Here's the drawing with two shaded views (mm, measured from the low corner). I have some questions. Coordinates: 2 decimals unless noted, no trailing zeros. Write each loop counter-clockwise with the first axis right and the second up, starting at its lowest first coordinate (ties: lowest second). Pieces come first, ordered by that corner, then holes. Notation, with made-up numbers: (42, 13) -> (99, 13) arc R26 ccw to (99, 27) -> close; hole circle Ø9 at (85.5, -2.5). An arc over 180 degrees is marked (long way). Use one line per item in the form item = value.
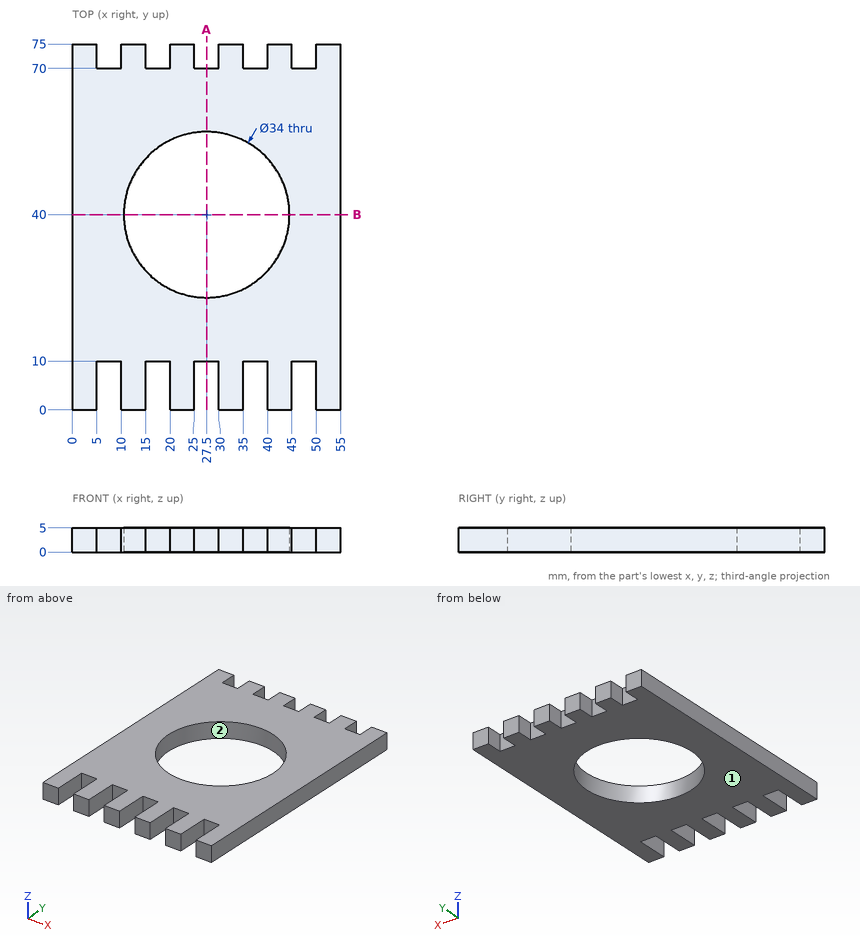
Q1. Suppose I cut it at B-B (y = 40). Write out the boundary of the cut face in (x, z), then the cut area to 3 significant figures.
Return value:
outline = (0, 0) -> (10.5, 0) -> (10.5, 5) -> (0, 5) -> close; (44.5, 0) -> (55, 0) -> (55, 5) -> (44.5, 5) -> close
area = 105 mm2
Q2. Will these pins go through, and if not, where does the flat tip stop? pin 1 (2.5 mm diameter, centred on x = 27, z = 1.5, fed in from -Y); pin 2 (2 mm diameter, centred on x = 38, z = 1, fed in from +Y).
Return value:
pin_1 = 10
pin_2 = 70
Q3. If I drill on line 1 (X direction, y = 7, z = 4.1); line 2 (Y direction, x = 27.5, z = 3.6); line 3 (X direction, y = 40.5, z = 4.2), over which ranges is the centre line in solid material (lowest first)? Write a range as from..to.
Return value:
line_1 = 0..5, 10..15, 20..25, 30..35, 40..45, 50..55
line_2 = 10..23, 57..70
line_3 = 0..10.51, 44.49..55
Q4. Suppose I cut it at A-A (x = 27.5). Write out the boundary of the cut face in (y, z).
Return value:
outline = (10, 0) -> (23, 0) -> (23, 5) -> (10, 5) -> close; (57, 0) -> (70, 0) -> (70, 5) -> (57, 5) -> close
Q5. Thinking about a two-plate mould opening in X: for the marked faces 1 and 2, which applies, released by +X, released by -X, zero draft, split by the parting line, or undercut?
Return value:
face_1 = zero draft
face_2 = undercut
